Verification items for this drawing (mm, ordinates from the low corner). A direction names the side the tool comes from. Round coordinates to 2 decimals unless told otherwise and drop trailing zeros. Write each loop counter-clockwise with the first axis right and the second up, starting at its lowest first coordinate (ties: lowest second). Pieces come first, ordered by that corner, then holes. Notation, with made-up numbers: M 33,20.25 L 78,20.25 A27 ccw 78,51.25 Z; hole C 34,-37 d10. An arc over 180 degrees is marked long. One line per question, with ' | ' between items. Start each with the question number.
Q1. Release check for a two-part mould opening along Y. For the marked faces 1, 2, 3 and 4 record: released by +Y, released by -Y, zero draft, split by the parting line, or undercut.
Q2. Gauge pin test, flat ends, axial feed: pin 1 (7 mm diameter, centred on y = 15, z = 9.5, fed in from +X); pin 2 (8 mm diameter, centred on y = 19, z = 24.5, fed in from -X) (1 decimal); pin 3 (12 mm diameter, centred on x = 39, z = 11, fed in from +Y); pin 4 (8 mm diameter, centred on x = 16.5, y = 19.5, fed in from +Z). Record the tip position at first contact, or that the pin passes through.
Q3. Cross-section at D-D (y = 18.5). Record the boundary of the cut face in (x, z).
Q4. Tool access check on the marked faces 5, 6, 7 and 8. Record the directions out of +Z, -Z, +X, -X, +Y, -Y that give a thin tool (end or side, any length) a straight path to the whole face; none if there is none.
Q5. Cross-section at B-B (x = 8). Record the boundary of the cut face in (y, z).
Q6. Thickness scan on line 1 along X through (y, z) = (18.5, 6.5); line 2 along Y through (x, z) = (8, 3.35); line 3 along X through (y, z) = (14.25, 21) (1 decimal). Record the ranges inside material, lowest first. Write a range as from..to.
Q7. Cross-section at A-A (y = 12.7). State how many separate pieces and enclosed holes the cut face has.
Q8. Cross-section at C-C (z = 21). Record the boundary of the cut face in (x, y) (1 decimal), then the cut area to 3 significant figures.
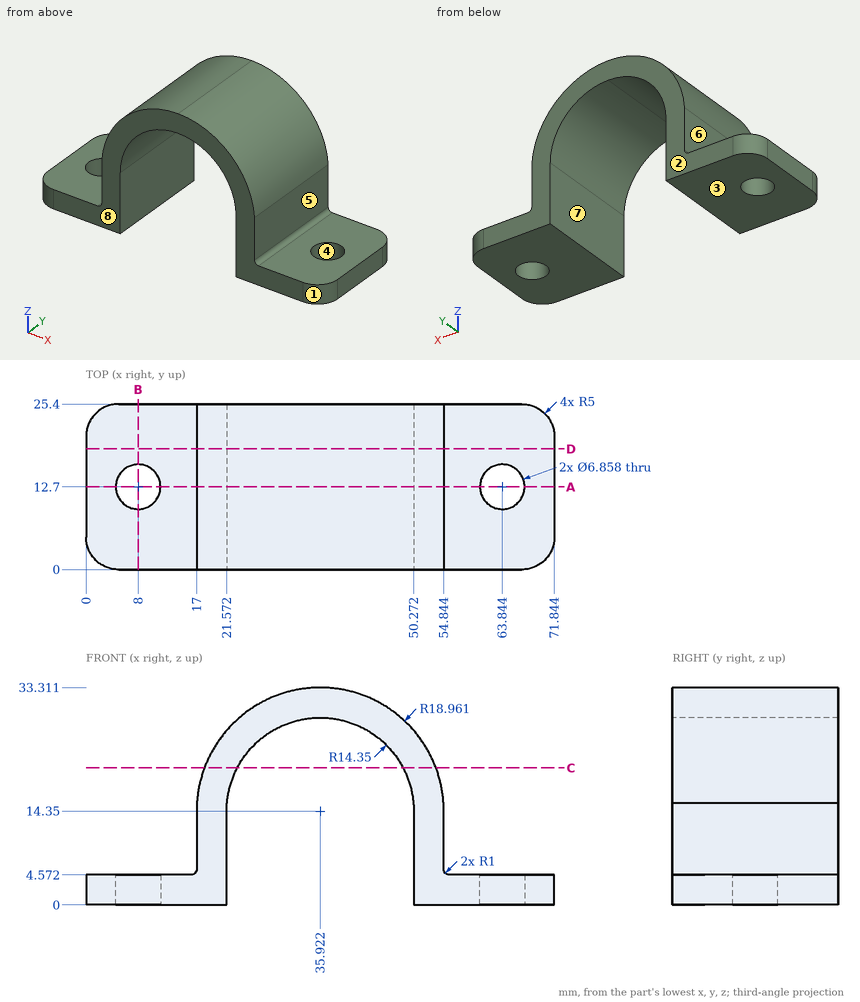
Determined:
1) face 1: released by -Y | face 2: released by +Y | face 3: zero draft | face 4: undercut
2) pin 1: stops at x = 54.84 | pin 2: stops at x = 18 | pin 3: passes through | pin 4: stops at z = 25.38
3) outline: M 0,0 L 21.57,0 L 21.57,14.35 A14.35 cw 50.27,14.35 L 50.27,0 L 71.84,0 L 71.84,4.57 L 55.84,4.57 A1 cw 54.84,5.57 L 54.84,15.57 A18.96 ccw 17,15.57 L 17,5.57 A1 cw 16,4.57 L 0,4.57 Z
4) face 5: +Z, +X, +Y, -Y | face 6: +Z, -X, +Y, -Y | face 7: -Z, +Y, -Y | face 8: +Z, -Z, +X, -X, -Y
5) outline: M 0,0 L 9.27,0 L 9.27,4.57 L 0,4.57 Z; M 16.13,0 L 25.4,0 L 25.4,4.57 L 16.13,4.57 Z
6) line 1: x = 17..21.57, 50.27..54.84 | line 2: y = 0..9.27, 16.13..25.4 | line 3: x = 18.2..23.2, 48.6..53.7
7) separate pieces: 3 | enclosed holes: 0
8) outline: M 18.2,0 L 23.2,0 L 23.2,25.4 L 18.2,25.4 Z; M 48.6,0 L 53.7,0 L 53.7,25.4 L 48.6,25.4 Z | area: 256 mm²
